```python
from build123d import *

# Parameters (mm, degrees)
SKETCH4_W          = 4.7625
SKETCH4_H          = 34.925
CUT_EXTRUDE1_DEPTH = 2.38125


with BuildPart() as part:
    # Sketch3 → Revolve2 (revolve)
    with BuildSketch(Plane(origin=(0, 0, 0), x_dir=(0, 0, -1), z_dir=(1, 0, 0)), mode=Mode.PRIVATE) as revolve2_sk:
        with BuildLine():
            Line((-186.95544175, 0), (-177.8, 0))
            Line((-177.8, 0), (0, 0))
            Line((0, 0), (0, 6.35))
            Line((0, 6.35), (-26.8925, 6.35))
            Line((-26.8925, 6.35), (-26.8925, 7.9375))
            Line((-26.8925, 7.9375), (-109.125, 7.9375))
            Line((-109.125, 7.9375), (-109.125, 8.73125))
            Line((-109.125, 8.73125), (-112.3, 8.73125))
            Line((-112.3, 8.73125), (-112.3, 6.109884817))
            Line((-112.3, 6.109884817), (-176.558072773, 4.689142192))
            ThreePointArc((-176.558072773, 4.689142192), (-176.816471065, 4.656721397), (-177.062823544, 4.572274718))
            Line((-177.062823544, 4.572274718), (-186.95544175, 0))
        make_face()
    revolve(revolve2_sk.sketch.rotate(Axis((0, 0, 0), (0, 0, 1)), 90), axis=Axis((0, 0, 0), (0, 0, 1)))

    # Sketch4 → Cut-Extrude1 (cut)
    with BuildSketch(Plane(origin=(0, 7.9375, 0), x_dir=(1, 0, 0), z_dir=(0, 1, 0))):
        with Locations((0, -62.855066403)):
            Rectangle(SKETCH4_W, SKETCH4_H)
    extrude(amount=-CUT_EXTRUDE1_DEPTH, mode=Mode.SUBTRACT)


solid = part.part
```
Geometry check sheet. Reference: the model listing, model coordinates, mm. A direction names the side the tool comes from. Give positions to 0.01 mm unless a question says otherwise; leave off trailing zeros. Write each loop counter-clockwise with the first axis right and the second up, starting at its lowest first coordinate (ties: lowest second). Pieces come first, ordered by that corner, then holes.
1) Section check A-A, the plane z = 84. Record the boundary of the cut face in (x, y) (1 decimal).
2) Section check B-B, the plane z = 156. Record the boundary of the cut face in (x, y).
3) Gauge pin test, flat ends, axial feed: pin 1 (8.5 mm diameter, centred on x = 2.5, y = -2.5, fed in from -Z); pin 2 (2 mm diameter, centred on y = 6.5, z = 64, fed in from -X); pin 3 (2 mm diameter, centred on x = 1, y = 0.5, fed in from +Z); pin 4 (2 mm diameter, centred on x = 7, z = 44, fed in from +Y). Record the tip position at first contact, or that the pin passes through.
4) Access from +Z, -Z, +X, -X, +Y, -Y to the whole of each face (thin tool, end or side, straight path). Record for faces 1 (the flat face through (-2, -6, 112.3)), 2 (the flat face through (0, -7, 26.892)), 3 (the flat face through (0, 0, 0)).
5) Material ranges on L1, parallel to Z at x = 6, y = 1.75; L2, parallel to Y at x = 1.75, z = 25; L3, parallel to Y at x = -0.5, z = 36.5, recorded low to high.
6) Release check for a two-part mould opening along X. For faces 4 (the cylindrical face through (5.04, 3.86, 13.63)), 5 (the flat face through (0, 5.556, 63)), 6 (the flat face through (2, 8, 109.125)) record: pulls with the +X half, pulls with the -X half, needs draft (parallel to the pull), parting line crosses it, or undercut.
Computed:
1. outline: circle Ø15.9 at (0, 0)
2. outline: circle Ø10.29 at (0, 0)
3. pin 1: stops at z = 0
3. pin 2: stops at x = -5.72
3. pin 3: stops at z = 186.7
3. pin 4: stops at y = 5.2
4. face 1: +Z
4. face 2: -Z
4. face 3: -Z, +X, -X, +Y, -Y
5. L1: z = 0 to 112.3
5. L2: y = -6.1 to 6.1
5. L3: y = -7.92 to 7.92
6. face 4: parting line crosses it
6. face 5: undercut
6. face 6: needs draft
